Check sheet for the modelled part. Datum: model origin and axes. Units: mm. A direction names the side the tool comes from. Coordinates: 2 decimals unless noted, no trailing zeros. Loops run counter-clockwise (first coordinate to the right, second up) from the corner with the lowest first, then second, coordinate; pieces in that order, holes last. Notation, with made-up numbers: (22.5, -30.5) -> (55.5, -30.5) arc R14 cw to (55.5, -7.5) -> close; hole circle Ø7 at (62, 2.25). An arc over 180 degrees is marked (long way). Use CSV: the item, a comma, the result in double quotes. Start each with the question number.
1. Set-up check for faces 5 (the face through (110, -29, 3)), 6 (the face through (-22, 31, 6)): record each of +Z, -Z, +X, -X, +Y, -Y from which the full face is reachable in a straight line by a thin tool's end or side.
2. Sectioned sample at B-B, the plane y = 3.5. Record the cut outline in (x, z), and give its area (3 significant figures).
3. Gauge pin test, flat ends, axial feed: pin 1 (3 mm diameter, centred on x = 120, z = 3, fed in from -Y); pin 2 (3 mm diameter, centred on y = -24, z = 2.5, fed in from +X); pin 3 (2.5 mm diameter, centred on y = -25, z = 3, fed in from +X); pin 4 (10 mm diameter, centred on x = -26.5, y = 23, fed in from +Z). Record the tip position at first contact, or that the pin passes through.
4. Sectioned sample at A-A, the plane x = -50. Record the cut outline in (y, z), and give its area (3 significant figures).
5. Sectioned sample at C-C, the plane z = 2.5. Count the separate pieces of the cut face and the enclosed holes in it, and give its area (3 significant figures).
6. Thickness scan on L1, parallel to Y at x = -142.8, z = 3; L2, parallel to X at y = -31.2, z = 3; L3, parallel to Y at x = 112, z = 4.8. Record the ranges inside material, lowest first.
7. Release check for a two-part mould opening along Y. For faces 1 (the face through (140, 0, 3)), 2 (the face through (-2, -35, 3)), 3 (the face through (103, 29, 3)), 4 (the face through (-146, 0, 3)) record: pulls with the +Y half, pulls with the -Y half, needs draft (parallel to the pull), parting line crosses it, or undercut.
```python
from build123d import *

# Parameters (mm, degrees)
SKETCH_1_W          = 292
SKETCH_1_H          = 70
SKETCH_1_W_2        = 280
SKETCH_1_H_2        = 58
EXTRUDE_1_DEPTH     = 6
EXTRUDE_2_DEPTH     = 6
SKETCH_3_R          = 2
CUT_EXTRUDE_1_DEPTH = 6
SKETCH_4_R          = 2
CUT_EXTRUDE_2_DEPTH = 6


with BuildPart() as part:
    # 草图1 → 凸台-拉伸1 (new body)
    with BuildSketch(Plane.XY):
        Rectangle(SKETCH_1_W, SKETCH_1_H)
        Rectangle(SKETCH_1_W_2, SKETCH_1_H_2, mode=Mode.SUBTRACT)
    extrude(amount=EXTRUDE_1_DEPTH)

    # 草图2 → 凸台-拉伸2 (add)
    with BuildSketch(Plane.XY):
        Polygon((-78.646881702, -29), (-81.752710243, -29), (-66.211657082, 29), (-60, 29), (-75.541053161, -29), align=None)
        Polygon((75.541053161, -29), (78.646881702, -29), (81.752710243, -29), (66.211657082, 29), (60, 29), align=None)
    extrude(amount=EXTRUDE_2_DEPTH)

    # 草图3 → 切除-拉伸1 (cut)
    with BuildSketch(Plane.ZY.offset(146)):
        with Locations((3, 25)):
            Circle(SKETCH_3_R)
        with Locations((3, -25)):
            Circle(SKETCH_3_R)
    cut_extrude_1 = extrude(amount=-CUT_EXTRUDE_1_DEPTH, mode=Mode.SUBTRACT)

    # 镜向1: 切除-拉伸1 across plane
    add(cut_extrude_1.mirror(Plane(origin=(0, 0, 0), x_dir=(0, 0, 1), z_dir=(1, 0, 0))), mode=Mode.SUBTRACT)

    # 草图4 → 切除-拉伸2 (cut)
    with BuildSketch(Plane.XZ.offset(35)):
        with Locations(Location((-120, 3, 0), (0, 0, 270))):
            Circle(SKETCH_4_R)
        with Locations(Location((-100, 3, 0), (0, 0, 270))):
            Circle(SKETCH_4_R)
        with Locations(Location((120, 3, 0), (0, 0, 90))):
            Circle(SKETCH_4_R)
        with Locations(Location((100, 3, 0), (0, 0, 90))):
            Circle(SKETCH_4_R)
    extrude(amount=-CUT_EXTRUDE_2_DEPTH, mode=Mode.SUBTRACT)


solid = part.part
```
Completed:
1,face 5,"+Z, -Z"
1,face 6,"+Z, +X, -X, +Y, -Y"
2,outline,"(-146, 0) -> (-140, 0) -> (-140, 6) -> (-146, 6) -> close; (-73.04, 0) -> (-66.83, 0) -> (-66.83, 6) -> (-73.04, 6) -> close; (66.83, 0) -> (73.04, 0) -> (73.04, 6) -> (66.83, 6) -> close; (140, 0) -> (146, 0) -> (146, 6) -> (140, 6) -> close"
2,area,"147 mm²"
3,pin 1,"y = 29"
3,pin 2,"x = 146"
3,pin 3,"x = 81.02"
3,pin 4,"through"
4,outline,"(-35, 0) -> (-29, 0) -> (-29, 6) -> (-35, 6) -> close; (29, 0) -> (35, 0) -> (35, 6) -> (29, 6) -> close"
4,area,"72.0 mm²"
5,separate pieces,"7"
5,enclosed holes,"1"
5,area,"4,730 mm²"
6,L1,"-35 to -27, -23 to 23, 27 to 35"
6,L2,"-146 to -122, -118 to -102, -98 to 98, 102 to 118, 122 to 146"
6,L3,"-35 to -29, 29 to 35"
7,face 1,"undercut"
7,face 2,"pulls with the -Y half"
7,face 3,"undercut"
7,face 4,"needs draft"
